from build123d import *

# Parameters (mm, degrees)
SKETCH1_W           = 65
SKETCH1_H           = 50
BOSS_EXTRUDE1_DEPTH = 150
SKETCH2_W           = 15
SKETCH2_H           = 50
BOSS_EXTRUDE2_DEPTH = 10
SKETCH3_R           = 5
BOSS_EXTRUDE3_DEPTH = 20
SKETCH4_W           = 65
SKETCH4_H           = 63
CUT_EXTRUDE1_DEPTH  = 183.225821441


with BuildPart() as part:
    # Sketch1 → Boss-Extrude1 (new body)
    with BuildSketch(Plane.XY):
        Rectangle(SKETCH1_W, SKETCH1_H)
    extrude(amount=BOSS_EXTRUDE1_DEPTH)

    # Sketch2 → Boss-Extrude2 (add)
    with BuildSketch(Plane(origin=(32.5, 0, 0), x_dir=(0, 0, -1), z_dir=(1, 0, 0))):
        with Locations((-75, 0)):
            Rectangle(SKETCH2_W, SKETCH2_H)
    boss_extrude2 = extrude(amount=BOSS_EXTRUDE2_DEPTH)

    # Mirror1: Boss-Extrude2 across plane
    add(boss_extrude2.mirror(Plane(origin=(0, 0, 0), x_dir=(0, 0, 1), z_dir=(1, 0, 0))))

    # Sketch3 → Boss-Extrude3 (add)
    with BuildSketch(Plane.XY.offset(150)):
        Circle(SKETCH3_R)
    extrude(amount=BOSS_EXTRUDE3_DEPTH)

    # Sketch4 → Cut-Extrude1 (cut, through all)
    with BuildSketch(Plane(origin=(0, 25, 0), x_dir=(1, 0, 0), z_dir=(0, 1, 0))):
        with Locations((0, -31.5)):
            Rectangle(SKETCH4_W, SKETCH4_H)
    extrude(amount=-CUT_EXTRUDE1_DEPTH, mode=Mode.SUBTRACT)


solid = part.part
Check sheet for the modelled part. Datum: model origin and axes. Units: mm. A direction names the side the tool comes from. Round coordinates to 2 decimals unless told otherwise and drop trailing zeros. Loops run counter-clockwise (first coordinate to the right, second up) from the corner with the lowest first, then second, coordinate; pieces in that order, holes last.
1. Sectioned sample at C-C on z = 108. Record the boundary of the cut face in (x, y).
2. Sectioned sample at A-A on x = 0. Record the boundary of the cut face in (y, z), and give its area (3 significant figures).
3. Sectioned sample at B-B on y = 8. Record the boundary of the cut face in (x, z), and give its area (4 significant figures).
4. Sectioned sample at D-D on y = 0. Record the boundary of the cut face in (x, z).
5. Gauge pin test, flat ends, axial feed: pin 1 Ø10 at (y, z) = (-15, 116.5) entering from +X; pin 2 Ø5 at (x, y) = (39, 4.5) entering from +Z; pin 3 Ø12 at (x, y) = (27, -11) entering from +Z. Record the tip position at first contact, or that the pin passes through.
6. Scan lines: probe 1 along Z at (x, y) = (13.5, -13); probe 2 along X at (y, z) = (1, 109); probe 3 along Z at (x, y) = (35, 17). Record each from-to range of solid material in increasing order.
7. Set-up check for faces 1 (the flat face through (-32.5, 0, 65)), 2 (the cylindrical face through (-1.08, -4.88, 159.86)), 3 (the flat face through (-32.5, 0, 116)): record each of +Z, -Z, +X, -X, +Y, -Y from which the full face is reachable in a straight line by a thin tool's end or side.
Recorded:
1. outline: (-32.5, -25) - (32.5, -25) - (32.5, 25) - (-32.5, 25) - close
2. outline: (-25, 63) - (25, 63) - (25, 150) - (5, 150) - (5, 170) - (-5, 170) - (-5, 150) - (-25, 150) - close
2. area: 4,550 mm2
3. outline: (-42.5, 67.5) - (-32.5, 67.5) - (-32.5, 63) - (32.5, 63) - (32.5, 67.5) - (42.5, 67.5) - (42.5, 82.5) - (32.5, 82.5) - (32.5, 150) - (-32.5, 150) - (-32.5, 82.5) - (-42.5, 82.5) - close
3. area: 5,955 mm2
4. outline: (-42.5, 67.5) - (-32.5, 67.5) - (-32.5, 63) - (32.5, 63) - (32.5, 67.5) - (42.5, 67.5) - (42.5, 82.5) - (32.5, 82.5) - (32.5, 150) - (5, 150) - (5, 170) - (-5, 170) - (-5, 150) - (-32.5, 150) - (-32.5, 82.5) - (-42.5, 82.5) - close
5. pin 1: stops at x = 32.5
5. pin 2: stops at z = 82.5
5. pin 3: stops at z = 150
6. probe 1: z = 63 to 150
6. probe 2: x = -32.5 to 32.5
6. probe 3: z = 67.5 to 82.5
7. face 1: -Z, -X, +Y, -Y
7. face 2: +Z
7. face 3: +Z, -X, +Y, -Y
